Here's how the part is built. I have some questions about the finished solid (model axes, mm). A direction names the side the tool comes from. Coordinates: 2 decimals unless noted, no trailing zeros. Order: outer loops, then holes, each group sorted by start corner. A loop starts at its lowest first (then second) coordinate and runs counter-clockwise, first axis right, second up.
```python
from build123d import *

# Parameters (mm, degrees)
SKETCH1_W           = 17.377025631
SKETCH1_H           = 16.239323069
BOSS_EXTRUDE1_DEPTH = 80
BOSS_EXTRUDE2_DEPTH = 80


with BuildPart() as part:
    # Sketch1 → Boss-Extrude1 (new body)
    with BuildSketch(Plane.XY):
        Polygon((-25.191985327, 24.243899858), (-82.889758174, 24.243899858), (-82.889758174, -23.756100142), (-74.789758174, -23.756100142), (-74.789758174, -3.629600036), (-65.986748664, -3.629600036), (-65.986748664, -23.756100142), (-25.191985327, -23.756100142), align=None)
        with Locations((-45.670631465, 5.119661535)):
            Rectangle(SKETCH1_W, SKETCH1_H, mode=Mode.SUBTRACT)
    extrude(amount=-BOSS_EXTRUDE1_DEPTH)

    # Sketch1_6 → Boss-Extrude2 (add)
    with BuildSketch(Plane.XY):
        Polygon((-54.040871751, 48.623240497), (-25.191985327, 24.243899858), (-82.889758174, 24.243899858), align=None)
    extrude(amount=-BOSS_EXTRUDE2_DEPTH)


solid = part.part
```
Q1. We'd pull the mould along X, two halves only. Please class faces 1 (the flat face through (-82.89, 1, -39)), 2 (the flat face through (-36.982, 5, -39)), 3 (the flat face through (-79, -23.756, -39)): pulls with the +X half, pulls with the -X half, needs draft (parallel to the pull), parting line crosses it, or undercut.
Q2. If we section it at A-A on y = 9.5: Write out the boundary of the cut face in (x, z).
Q3. If we section it at C-C on x = -44.5: Write out the boundary of the cut face in (y, z), then the cut area to 3 significant figures.
Q4. Will this pin go through, and if not, where does the flat tip stop? pin 1 (14 mm diameter, centred on x = -44, z = -42, fed in from +Y).
Q5. If we section it at B-B on z = -65: Write out the boundary of the cut face in (x, y), then the cut area to 3 significant figures.
Q6. I need wall thicknesses on L1, parallel to X at y = -10.5, z = -39.5; L2, parallel to X at y = 4.5, z = -27.5; L3, parallel to Y at x = -45, z = -36.5. Which ranges of each line are inside material? Lowest first, please.
Q7. If we section it at D-D on y = 26: Write out the boundary of the cut face in (x, z).
Q8. For faces 4 (the flat face through (-65.987, -14, -39)), 5 (the flat face through (-60, 5, 0)), 6 (the flat face through (-54.359, 5, -39)), which set-ups out of +Z, -Z, +X, -X, +Y, -Y let a thin tool reach every point of the face, with its end or its side?
Reply:
1. face 1: pulls with the -X half
1. face 2: undercut
1. face 3: needs draft
2. outline: (-82.89, -80) - (-54.36, -80) - (-54.36, 0) - (-82.89, 0) - close; (-36.98, -80) - (-25.19, -80) - (-25.19, 0) - (-36.98, 0) - close
3. outline: (-23.76, -80) - (-3, -80) - (-3, 0) - (-23.76, 0) - close; (13.24, -80) - (40.56, -80) - (40.56, 0) - (13.24, 0) - close
3. area: 3,850 mm2
4. pin 1: stops at y = 46.05
5. outline: (-82.89, -23.76) - (-74.79, -23.76) - (-74.79, -3.63) - (-65.99, -3.63) - (-65.99, -23.76) - (-25.19, -23.76) - (-25.19, 24.24) - (-54.04, 48.62) - (-82.89, 24.24) - close; hole (-54.36, -3) - (-36.98, -3) - (-36.98, 13.24) - (-54.36, 13.24) - close
5. area: 3,010 mm2
6. L1: x = -82.89 to -74.79, -65.99 to -25.19
6. L2: x = -82.89 to -54.36, -36.98 to -25.19
6. L3: y = -23.76 to -3, 13.24 to 40.98
7. outline: (-80.81, -80) - (-27.27, -80) - (-27.27, 0) - (-80.81, 0) - close
8. face 4: +Z, -Z, -Y
8. face 5: +Z, +X, -X, +Y, -Y
8. face 6: +Z, -Z
